Source: CAD feature listing. Evaluate the final solid. Frame: model axes, mm. A direction names the side the tool comes from. Give positions to 0.01 mm unless a question says otherwise; leave off trailing zeros. Write each loop counter-clockwise with the first axis right and the second up, starting at its lowest first coordinate (ties: lowest second). Pieces come first, ordered by that corner, then holes. Notation, with made-up numbers: (-40, 9.25) -> (1, 9.25) arc R9 ccw to (1, 25.25) -> close; hole circle Ø11 at (-36.5, -8). An arc over 180 degrees is marked (long way). Write item = value, one per line.
Autodesk Inventor part; units mm, degrees
ref_plane "YZ Plane" through (0, 0, 0) normal (1, 0, 0) x (0, 1, 0)
ref_plane "XZ Plane" through (0, 0, 0) normal (0, 1, 0) x (-1, 0, 0)
ref_plane "XY Plane" through (0, 0, 0) normal (0, 0, 1) x (1, 0, 0)
sketch "Sketch1" plane through (0, 0, 0) normal (0, 0, 1) x (1, 0, 0)
  line L0 (-50, -110) -> (50, -110)
  line L1 (50, -110) -> (50, 110)
  line L2 (50, 110) -> (-50, 110)
  line L3 (-50, 110) -> (-50, -110)
  line L4 (-50, -110) -> (50, 110) construction
  line L5 (50, -110) -> (-50, 110) construction
  point P0 (0, 0)
  dimension "d0" = 100
  dimension "d1" = 220
extrude "Extrusion1" add sketch "Sketch1" along normal blind 5
sketch "Sketch2" plane through (-50, 110, 0) normal (0, 1, 0) x (1, 0, 0)
  line L0 (0, 0) -> (100, 0)
  line L1 (0, 0) -> (49.9986, 49.9986)
  line L2 (49.9986, 49.9986) -> (53.5341, 46.463)
  line L3 (53.5341, 46.463) -> (3.5355, -3.5355)
  line L4 (3.5355, -3.5355) -> (0, 0)
  line L5 (0, 0) -> (70.7086, 0) construction
  line L6 (100.108, -0.1109) -> (53.5341, 46.463)
  line L7 (53.5341, 46.463) -> (49.9986, 42.9275)
  line L8 (49.9986, 42.9275) -> (96.5724, -3.6464)
  line L9 (96.5724, -3.6464) -> (100.108, -0.1109)
  point P0 (50, 0)
  point P1 (49.9986, 42.9275)
  dimension "d4" = 45
  dimension "d5" = 5
  dimension "d6" = 5
extrude "Extrusion2" add sketch "Sketch2" against normal blind 45 contours L1 L2 L3 L0 | L0 L3 L4 | L8 L3 L6 L0 | L0 L6 L9 L8
sketch "Sketch5" plane through (0, 0, 5) normal (0, 0, 1) x (1, 0, 0)
  line L0 (4.9986, 85) -> (-5.0014, 85)
  line L1 (-25.0014, 65) -> (-25.0014, 55)
  line L2 (-5.0014, 35) -> (4.9986, 35)
  line L3 (24.9986, 55) -> (24.9986, 65)
  line L4 (-0.0014, 110) -> (-0.0014, 65)
  line L5 (24.9986, 85) -> (-25.0014, 35) construction
  line L6 (-25.0014, 85) -> (24.9986, 35) construction
  arc A0 (4.9986, 35) -> (24.9986, 55) centre (4.9986, 55) ccw
  arc A1 (-25.0014, 55) -> (-5.0014, 35) centre (-5.0014, 55) ccw
  arc A2 (-5.0014, 85) -> (-25.0014, 65) centre (-5.0014, 65) ccw
  arc A3 (24.9986, 65) -> (4.9986, 85) centre (4.9986, 65) ccw
  point P0 (0, 0)
  point P1 (-0.0014, 60)
  dimension "d16" = 50
  dimension "d17" = 50
  dimension "d18" = 20
extrude "Extrusion5" cut sketch "Sketch5" against normal blind 5
properties part number "fixation_v04"
1) Draft query along X for faces 6 (the flat face through (21.162, 87.815, -21.764)), 7 (the flat face through (50, -2, 2)), 8 (the flat face through (0, 110, 2)), 9 (the flat face through (-50, 2, 2)). Return one class per face: pulls with the +X half, pulls with the -X half, needs draft (parallel to the pull), parting line crosses it, or undercut.
Computed:
face_6 = undercut
face_7 = pulls with the +X half
face_8 = needs draft
face_9 = pulls with the -X half
2) Cut plane A-A (y = 59.5). Return the cut outline in (x, z).
Computed:
outline = (-50, 0) -> (-25, 0) -> (-25, 5) -> (-50, 5) -> close; (25, 0) -> (50, 0) -> (50, 5) -> (25, 5) -> close
3) Material intervals for L1, parallel to Z at x = 40, y = -13.5; L2, parallel to Y at x = -8.5, z = 3.5; L3, parallel to X at y = 99.5, z = -34.5, sorted ascending.
Computed:
L1 = 0 to 5
L2 = -110 to 35.31, 84.69 to 110
L3 = -15.5 to -8.43, 8.43 to 15.5
4) Cut plane B-B (x = -31). Return the cut outline in (y, z), then the cut area to 3 significant figures.
Computed:
outline = (-110, 0) -> (110, 0) -> (110, 5) -> (-110, 5) -> close; (65, -19) -> (110, -19) -> (110, -11.93) -> (65, -11.93) -> close
area = 1,420 mm²
5) Cut plane D-D (y = -65.5). Return the cut outline in (x, z).
Computed:
outline = (-50, 0) -> (50, 0) -> (50, 5) -> (-50, 5) -> close
6) Contact query for flat-ended pins moving along their axis: pin 1 (1 mm diameter, centred on x = 21, y = 3.5, fed in from -Z); pin 2 (25 mm diameter, centred on x = -5.5, z = -30.5, fed in from -Y); pin 3 (5.5 mm diameter, centred on y = 6, z = 3.5, fed in from +X). Output: stop coordinate, or through.
Computed:
pin_1 = 0
pin_2 = 65
pin_3 = 50
7) Access query for faces 1 (the flat face through (0, 85, 3)), 2 (the flat face through (-11, 65, -33)), 3 (the flat face through (-21.165, 87.815, -21.764)), 4 (the flat face through (-1, -23, 0)), 5 (the cylindrical face through (-19.298, 41.014, 2.535)). Directions: +Z, -Z, +X, -X, +Y, -Y. A direction counts if a zero-diameter tool reaches every point of the face in a straight line with its end or side. Return the directions, or none.
Computed:
face_1 = +Z
face_2 = -Z, +X, -X, -Y
face_3 = +Y, -Y
face_4 = -Y
face_5 = +Z, -Z
8) Cut plane C-C (x = -17.5). Return the cut outline in (y, z), then the cut area to 3 significant figures.
Computed:
outline = (-110, 0) -> (39.39, 0) -> (39.39, 5) -> (-110, 5) -> close; (65, -32.5) -> (110, -32.5) -> (110, -25.43) -> (65, -25.43) -> close; (80.61, 0) -> (110, 0) -> (110, 5) -> (80.61, 5) -> close
area = 1,210 mm²
